Model file for the job. Use its own axes, mm. Face numbers are marked on the shaded views. A direction names the side the tool comes from. Give positions to 0.01 mm unless a question says otherwise; leave off trailing zeros. Loops run counter-clockwise (first coordinate to the right, second up) from the corner with the lowest first, then second, coordinate; pieces in that order, holes last. Notation, with made-up numbers: (18, 51.5) -> (54, 51.5) arc R24 ccw to (54, 83.5) -> close; hole circle Ø11 at (39.25, 1.5). An arc over 180 degrees is marked (long way). Use CSV: the item, a comma, the result in double quotes. Start each with the question number.
(1) Cut at B-B on z = 1.65. Write the cut outline in (x, y).
(2) Cut at C-C on x = 12. Write the cut outline in (y, z).
(3) Drill centre lines: probe 1 along X at (y, z) = (-3.5, 3.2); probe 2 along X at (y, z) = (0.25, 2.55); probe 3 along Y at (x, z) = (-11, 1.95). Where is each one in solid material? Low to high.
(4) 3-axis set-ups, long thin cutter, end or side, ignore diameter. For the marked faces 1 and 2: which of +Z, -Z, +X, -X, +Y, -Y reach the whole face in a straight line?
(5) Cut at A-A on y = -4.25. Write the cut outline in (x, z).
(6) Pull direction X, two halves, no side cores. Call the marked faces 3, 4 and 5: pulls with the +X half, pulls with the -X half, needs draft (parallel to the pull), parting line crosses it, or undercut.
from build123d import *

# Parameters (mm, degrees)
F0_W     = 21.924
F0_H     = 6.35
F1_DEPTH = 4


with BuildPart() as f1:
    # F0 (on Top) → F1 (new body)
    with BuildSketch(Plane.XY):
        with BuildLine():
            ThreePointArc((-15.281758, 0), (-12.781758, 2.5), (-10.281758, 0))
            Line((-10.281758, 0), (11.642242, 0))
            ThreePointArc((11.642242, 0), (14.142242, 2.5), (16.642242, 0))
            Line((16.642242, 0), (16.642242, -6.35))
            Line((16.642242, -6.35), (19.05, -6.35))
            Line((19.05, -6.35), (19.05, 6.35))
            Line((19.05, 6.35), (-19.05, 6.35))
            Line((-19.05, 6.35), (-19.05, -6.35))
            Line((-19.05, -6.35), (-15.281758, -6.35))
            Line((-15.281758, -6.35), (-15.281758, 0))
        make_face()
        with Locations((0.680242, -3.175)):
            Rectangle(F0_W, F0_H)
    extrude(amount=F1_DEPTH)


solid = f1.part
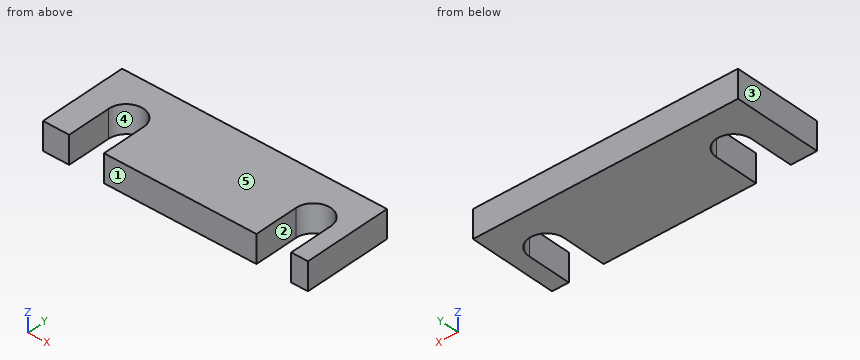
Check result:
1,outline,"(-19.05, -6.35) -> (-15.28, -6.35) -> (-15.28, 0) arc R2.5 cw to (-10.28, 0) -> (-10.28, -6.35) -> (11.64, -6.35) -> (11.64, 0) arc R2.5 cw to (16.64, 0) -> (16.64, -6.35) -> (19.05, -6.35) -> (19.05, 6.35) -> (-19.05, 6.35) -> close"
2,outline,"(1.29, 0) -> (6.35, 0) -> (6.35, 4) -> (1.29, 4) -> close"
3,probe 1,"-19.05 to -15.28, -10.28 to 11.64, 16.64 to 19.05"
3,probe 2,"-19.05 to -15.27, -10.29 to 11.65, 16.63 to 19.05"
3,probe 3,"1.75 to 6.35"
4,face 1,"+Z, -Z, +X, -X, -Y"
4,face 2,"+Z, -Z, -Y"
5,outline,"(-19.05, 0) -> (-15.28, 0) -> (-15.28, 4) -> (-19.05, 4) -> close; (-10.28, 0) -> (11.64, 0) -> (11.64, 4) -> (-10.28, 4) -> close; (16.64, 0) -> (19.05, 0) -> (19.05, 4) -> (16.64, 4) -> close"
6,face 3,"pulls with the -X half"
6,face 4,"undercut"
6,face 5,"needs draft"
